Build history of the part. All positions in model axes, mm. Face numbers are marked on the shaded views. Coordinates: 2 decimals unless noted, no trailing zeros. Write each loop counter-clockwise with the first axis right and the second up, starting at its lowest first coordinate (ties: lowest second). Pieces come first, ordered by that corner, then holes. Notation, with made-up numbers: (-3.5, 42.25) -> (44.5, 42.25) arc R33 cw to (44.5, 70.25) -> close; hole circle Ø3 at (14.25, 56.5). An arc over 180 degrees is marked (long way). Write each question's results on one line, items separated by ' | '. Start each with the question number.
Q1. Saw through at A-A on z = 1.25. Give the cut face in (x, y) (3 decimals).
Q2. Drill centre lines: line 1 (Y direction, x = 7, z = 6.25); line 2 (Y direction, x = -2.5, z = 0.5); line 3 (X direction, y = 2.75, z = -4.5). Where is each one in solid material? Low to high.
Q3. Saw through at C-C on z = 4.5. Give the cut face in (x, y) (3 decimals).
Q4. Two-plate mould, pull along X, no slides. Class the marked faces 1 and 2: released by +X, released by -X, zero draft, split by the parting line, or undercut.
Q5. Saw through at B-B on x = 36. Give the cut face in (y, z), and give its area (3 significant figures).
Q6. Drop flat-ended pins along their axis: pin 1 Ø8 at (x, y) = (27.5, 4) entering from -Z; pin 2 Ø2 at (x, z) = (-2.5, -1) entering from -Y; pin 3 Ø1.6 at (x, z) = (10.5, 0) entering from -Y; pin 4 Ø1 at (x, z) = (1.5, 6) entering from -Y. Give the stop position or say it passes through.
from build123d import *

# Parameters (mm, degrees)
F1_DEPTH = 8
F2_DEPTH = 2


with BuildPart() as f1:
    # F0 (on Top) → F1 (new body, symmetric)
    with BuildSketch(Plane.XY):
        with BuildLine():
            ThreePointArc((-7.5566905663, 5.7984526113), (2.5833573647, 9.1679817695), (9.4723611101, 1))
            Line((9.4723611101, 1), (11.4564392374, 1))
            ThreePointArc((11.4564392374, 1), (11.0364450387, 3.2321635028), (10.1859294227, 5.3382433249))
            ThreePointArc((10.1859294227, 5.3382433249), (8.2074300514, 8.055314516), (5.5278432783, 10.084292176))
            ThreePointArc((5.5278432783, 10.084292176), (-2.3684064244, 11.2534728421), (-9.1235634133, 7.0007564336))
            Line((-9.1235634133, 7.0007564336), (-7.5566905663, 5.7984526113))
        make_face()
    extrude(amount=F1_DEPTH, both=True)

    # F0 (on Top) → F2 (join)
    with BuildSketch(Plane.XY):
        with BuildLine():
            ThreePointArc((5.5278432783, 10.084292176), (8.2074300514, 8.055314516), (10.1859294227, 5.3382433249))
            Line((10.1859294227, 5.3382433249), (19.924339628, 0))
            Line((19.924339628, 0), (21.924339628, 1.0963274728))
            Line((21.924339628, 1.0963274728), (5.5278432783, 10.084292176))
        make_face()
        Polygon((21.924339628, 1.0963274728), (19.924339628, 0), (21.924339628, -1.0963274728), (23.924339628, 0), align=None)
        Polygon((23.924339628, 0), (21.924339628, -1.0963274728), (45.4999829336, -14.0196401956), (46.4242037672, -12.3336095953), align=None)
    extrude(amount=F2_DEPTH)


solid = f1.part
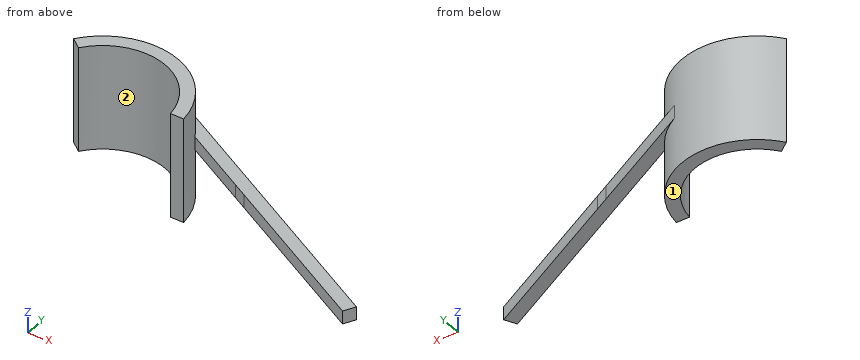
Returned:
1) outline: (-9.124, 7.001) -> (-7.557, 5.798) arc R9.525 cw to (9.472, 1) -> (11.456, 1) arc R11.5 ccw to (10.186, 5.338) -> (45.5, -14.02) -> (46.424, -12.334) -> (5.528, 10.084) arc R11.5 ccw to start
2) line 1: y = 6.46 to 9.12 | line 2: y = 9.19 to 11.22 | line 3: x = 9.12 to 11.17
3) outline: (-9.124, 7.001) -> (-7.557, 5.798) arc R9.525 cw to (9.472, 1) -> (11.456, 1) arc R11.5 ccw to start
4) face 1: zero draft | face 2: undercut
5) outline: (-8.81, 0) -> (-6.62, 0) -> (-6.62, 2) -> (-8.81, 2) -> close | area: 4.39 mm2
6) pin 1: passes through | pin 2: stops at y = 8.86 | pin 3: stops at y = 1 | pin 4: stops at y = 9.31
